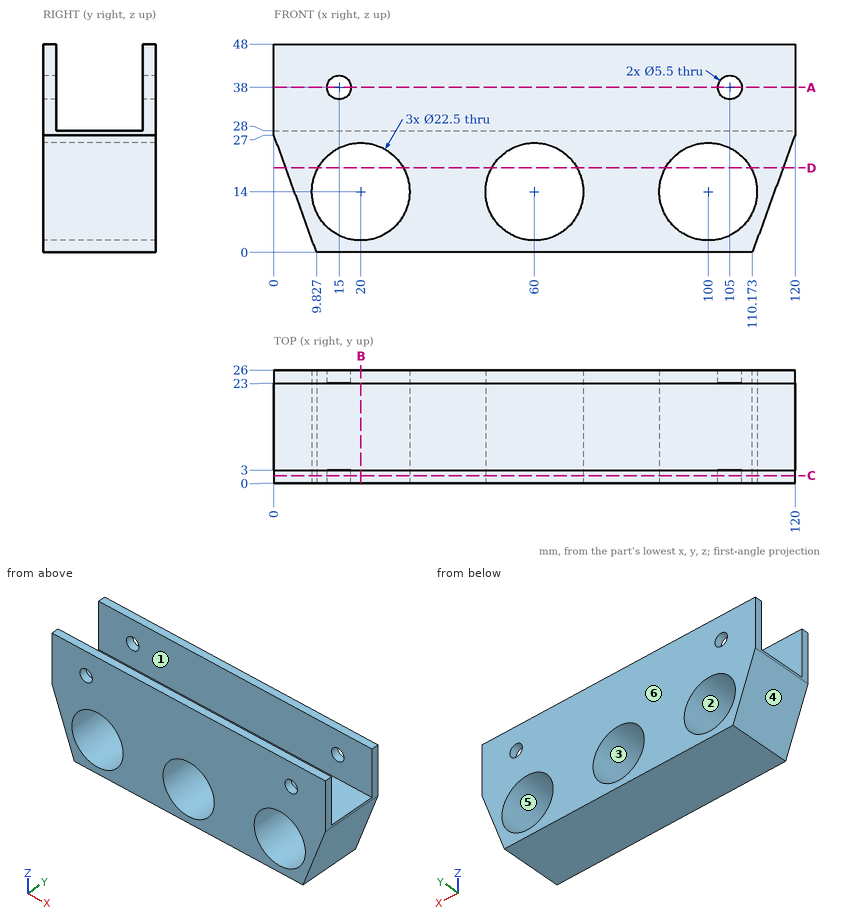
Study the drawing (mm; zero at the part's minimum x, y, z) and answer. A direction names the side the tool comes from. Give positions to 0.01 mm unless a question says otherwise; leave off trailing zeros. Loops run counter-clockwise (first coordinate to the right, second up) from the corner with the lowest first, then second, coordinate; pieces in that order, holes last. Notation, with made-up numbers: M -14,-6 L 19,-6 A18 ccw 19,1 Z; hole C -11.5,5 d11. An arc over 180 degrees is marked long. One line per item, written item: value. Start each with the question number.
1. Which of the six approach directions +Z, -Z, +X, -X, +Y, -Y give full straight-line access (tool end or side, diameter ignored) to the marked faces 1 and 2?
2. Find section D-D (z = 19.5). Give the vertices of the cut face in (x, y).
3. Find section C-C (y = 1.75). Give the vertices of the cut face in (x, z), and give its area (3 significant figures).
4. Find the intervals of material crossed by probe 1 along X at (y, z) = (2.1, 38); probe 2 along Z at (x, y) = (20, 17); probe 3 along X at (y, z) = (17.5, 14), in increasing order.
5. Determine the mould class of the marked faces 3, 4, 5 and 6 for opening direction Z: released by +Z, released by -Z, zero draft, split by the parting line, or undercut.
6. Find section A-A (z = 38). Give the vertices of the cut face in (x, y), and give its area (3 significant figures).
7. Each of these flat-tipped pins is pushed along its axis until it touches: P1, Ø16, axis at x = 85, z = 36, coming from the -Y side; P2, Ø1.5, axis at x = 92.5, y = 17, coming from the +Z side; P3, Ø4, axis at y = 7.5, z = 10, coming from the -X side; P4, Ø5, axis at y = 3, z = 19, coming from the -X side. Where does it stop, or does it pass through?
8. Find section B-B (x = 20). Give the vertices of the cut face in (y, z), and give its area (3 significant figures).
Reported:
1. face 1: +Z, +X, -X
1. face 2: +Y, -Y
2. outline: M 2.73,0 L 10.19,0 L 10.19,26 L 2.73,26 Z; M 29.81,0 L 50.19,0 L 50.19,26 L 29.81,26 Z; M 69.81,0 L 90.19,0 L 90.19,26 L 69.81,26 Z; M 109.81,0 L 117.27,0 L 117.27,26 L 109.81,26 Z
3. outline: M 0,27 L 9.83,0 L 110.17,0 L 120,27 L 120,48 L 0,48 Z; hole C 20,14 d22.5; hole C 15,38 d5.5; hole C 60,14 d22.5; hole C 100,14 d22.5; hole C 105,38 d5.5
3. area: 4,250 mm²
4. probe 1: x = 0 to 12.25, 17.75 to 102.25, 107.75 to 120
4. probe 2: z = 0 to 2.75, 25.25 to 28
4. probe 3: x = 4.73 to 8.75, 31.25 to 48.75, 71.25 to 88.75, 111.25 to 115.27
5. face 3: undercut
5. face 4: released by -Z
5. face 5: undercut
5. face 6: zero draft
6. outline: M 0,0 L 12.25,0 L 12.25,3 L 0,3 Z; M 0,23 L 12.25,23 L 12.25,26 L 0,26 Z; M 17.75,0 L 102.25,0 L 102.25,3 L 17.75,3 Z; M 17.75,23 L 102.25,23 L 102.25,26 L 17.75,26 Z; M 107.75,0 L 120,0 L 120,3 L 107.75,3 Z; M 107.75,23 L 120,23 L 120,26 L 107.75,26 Z
6. area: 654 mm²
7. P1: stops at y = 0
7. P2: stops at z = 28
7. P3: stops at x = 5.46
7. P4: stops at x = 2
8. outline: M 0,0 L 26,0 L 26,2.75 L 0,2.75 Z; M 0,25.25 L 26,25.25 L 26,48 L 23,48 L 23,28 L 3,28 L 3,48 L 0,48 Z
8. area: 263 mm²
